```python
from build123d import *

# Parameters (mm, degrees)
SKETCH1_W           = 38.5
SKETCH1_H           = 38.2
BOSS_EXTRUDE1_DEPTH = 32.7
SKETCH2_R           = 14.85
BOSS_EXTRUDE2_DEPTH = 52.6
SKETCH3_R           = 3.175
CUT_EXTRUDE1_DEPTH  = 7.2136
SKETCH4_R           = 2.06599734
BOSS_EXTRUDE3_DEPTH = 5.08


with BuildPart() as part:
    # Sketch1 → Boss-Extrude1 (new body)
    with BuildSketch(Plane.XY):
        Rectangle(SKETCH1_W, SKETCH1_H)
    extrude(amount=BOSS_EXTRUDE1_DEPTH)

    # Sketch2 → Boss-Extrude2 (add)
    with BuildSketch(Plane.XY.offset(32.7)):
        Circle(SKETCH2_R)
    extrude(amount=BOSS_EXTRUDE2_DEPTH)

    # Sketch3 → Cut-Extrude1 (cut)
    with BuildSketch(Plane(origin=(19.25, 0, 0), x_dir=(0, 0, -1), z_dir=(1, 0, 0))):
        with Locations((-7.554319607, 0)):
            Circle(SKETCH3_R)
    cut_extrude1 = extrude(amount=-CUT_EXTRUDE1_DEPTH, mode=Mode.SUBTRACT)

    # Mirror1: Cut-Extrude1 across plane
    add(cut_extrude1.mirror(Plane(origin=(0, 0, 0), x_dir=(0, 0, 1), z_dir=(1, 0, 0))), mode=Mode.SUBTRACT)

    # Sketch4 → Boss-Extrude3 (add)
    with BuildSketch(Plane(origin=(0, 0, 0), x_dir=(-1, 0, 0), z_dir=(0, 0, -1))):
        with Locations((0, -16.651600327)):
            Circle(SKETCH4_R)
    extrude(amount=BOSS_EXTRUDE3_DEPTH)


solid = part.part
```
Model file for the job. Use its own axes, mm. A direction names the side the tool comes from. Give positions to 0.01 mm unless a question says otherwise; leave off trailing zeros. Write each loop counter-clockwise with the first axis right and the second up, starting at its lowest first coordinate (ties: lowest second). Pieces come first, ordered by that corner, then holes. Notation, with made-up numbers: (-1.75, 11.5) - (53.25, 11.5) arc R22 ccw to (53.25, 42.5) - close; hole circle Ø2 at (25, -9). An arc over 180 degrees is marked (long way). One line per question, with ' | ' between items. Start each with the question number.
(1) 3-axis set-ups, long thin cutter, end or side, ignore diameter. For faces 1 (the face through (0, -17, -5.08)), 2 (the face through (0.45, -18.67, -2.5)), 3 (the face through (-15.694, 0.954, 4.526)), 4 (the face through (-9, 13, 32.7)), 5 (the face through (12.036, 0, 8)): which of +Z, -Z, +X, -X, +Y, -Y reach the whole face in a straight line?
(2) Slice it at D-D on z = 6.5. Write the cut outline in (x, y).
(3) Slice it at A-A on y = 0. Write the cut outline in (x, z).
(4) Wall check: line 1 along Z through (x, y) = (-16.5, -7); line 2 along Z through (x, y) = (-6, 12); line 3 along Y through (x, z) = (13.5, 69.5). Give the ranges that are in metal, low to high. Write a range as from..to.
(5) Slice it at C-C on x = 16.5. Write the cut outline in (y, z) (3 decimals).
(6) Pin check, flat tips, straight feed: P1, Ø5, axis at y = 0, z = 7.55, coming from the -X side; P2, Ø5, axis at y = -13, z = 61, coming from the +X side; P3, Ø6, axis at y = -14, z = 37, coming from the -X side. Stop position of each tip, or through.
(7) Two-plate mould, pull along Z, no slides. Class faces 6 (the face through (-11.78, -9.04, 58.63)), 7 (the face through (15.694, 0.954, 4.526)), 8 (the face through (0, 0, 0)): +Z half, -Z half, draft (parallel to the pull), parting line (faces both ways), or undercut.
(8) Slice it at B-B on x = 0. Write the cut outline in (y, z), plus the area to 3 significant figures.
Results below:
1) face 1: -Z, +X, -X, +Y, -Y | face 2: -Z | face 3: -X | face 4: +Z | face 5: +X
2) outline: (-19.25, -19.1) - (19.25, -19.1) - (19.25, -2.99) - (12.04, -2.99) - (12.04, 2.99) - (19.25, 2.99) - (19.25, 19.1) - (-19.25, 19.1) - (-19.25, 2.99) - (-12.04, 2.99) - (-12.04, -2.99) - (-19.25, -2.99) - close
3) outline: (-19.25, 0) - (19.25, 0) - (19.25, 4.38) - (12.04, 4.38) - (12.04, 10.73) - (19.25, 10.73) - (19.25, 32.7) - (14.85, 32.7) - (14.85, 85.3) - (-14.85, 85.3) - (-14.85, 32.7) - (-19.25, 32.7) - (-19.25, 10.73) - (-12.04, 10.73) - (-12.04, 4.38) - (-19.25, 4.38) - close
4) line 1: 0..32.7 | line 2: 0..85.3 | line 3: -6.19..6.19
5) outline: (-19.1, 0) - (19.1, 0) - (19.1, 32.7) - (-19.1, 32.7) - close; hole circle Ø6.35 at (0, 7.554)
6) P1: x = -12.04 | P2: x = 10.5 | P3: x = -9.98
7) face 6: draft | face 7: undercut | face 8: -Z half
8) outline: (-19.1, 0) - (-18.72, 0) - (-18.72, -5.08) - (-14.59, -5.08) - (-14.59, 0) - (19.1, 0) - (19.1, 32.7) - (14.85, 32.7) - (14.85, 85.3) - (-14.85, 85.3) - (-14.85, 32.7) - (-19.1, 32.7) - close | area: 2,830 mm^2
